Geometry check sheet. Reference: the model listing, model coordinates, mm. Coordinates: 2 decimals unless noted, no trailing zeros. Write each loop counter-clockwise with the first axis right and the second up, starting at its lowest first coordinate (ties: lowest second). Pieces come first, ordered by that corner, then holes. Notation, with made-up numbers: (35, 63) -> (76, 63) arc R17 cw to (76, 84) -> close; hole circle Ø7 at (20, 56). An arc over 180 degrees is marked (long way). Answer in a Markdown table with one row per item. Add a question column.
1. Cross-section at B-B on x = 17.5. Record the cut outline in (y, z), and give its area (3 significant figures).
2. Depth check by flat-ended pin: P1, Ø1.6, axis at x = 17.5, y = -52.5, coming from the -Z side. Enter the tip coordinate at first touch or a pass-through.
3. Scan line: L1, parallel to Y at x = 7.5, z = 6. Record every from-to range of solid material in increasing order. Write a range as from..to.
4. Cross-section at A-A on y = -7.5. Record the cut outline in (x, z), and give its area (3 significant figures).
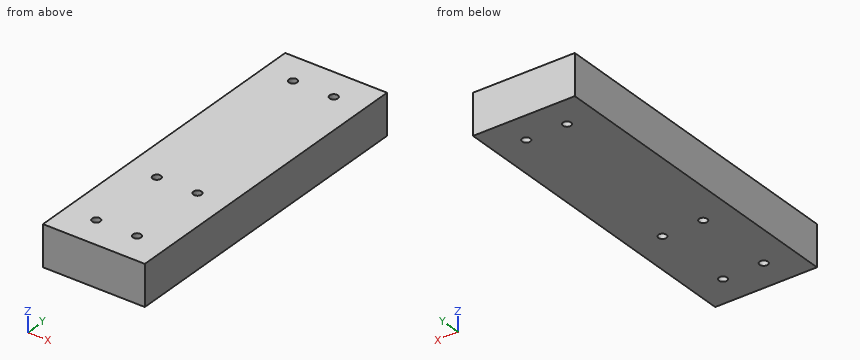
```python
from build123d import *

# Parameters (mm, degrees)
SKETCH1_W           = 25
SKETCH1_H           = 80
BOSS_EXTRUDE1_DEPTH = 10
SKETCH2_R           = 1
CUT_EXTRUDE1_DEPTH  = 85.409715081


with BuildPart() as part:
    # Sketch1 → Boss-Extrude1 (new body)
    with BuildSketch(Plane.XY):
        with Locations((12.5, -40)):
            Rectangle(SKETCH1_W, SKETCH1_H)
    extrude(amount=BOSS_EXTRUDE1_DEPTH)

    # Sketch2 → Cut-Extrude1 (cut, through all)
    with BuildSketch(Plane.XY.offset(10)):
        with Locations((7.5, -52.5)):
            Circle(SKETCH2_R)
        with Locations((7.5, -72.5)):
            Circle(SKETCH2_R)
        with Locations((7.5, -7.5)):
            Circle(SKETCH2_R)
        with Locations(Location((17.5, -7.5, 0), (0, 0, 180))):
            Circle(SKETCH2_R)
        with Locations(Location((17.5, -52.5, 0), (0, 0, 180))):
            Circle(SKETCH2_R)
        with Locations(Location((17.5, -72.5, 0), (0, 0, 180))):
            Circle(SKETCH2_R)
    extrude(amount=-CUT_EXTRUDE1_DEPTH, mode=Mode.SUBTRACT)


solid = part.part
```
Results found:
| question | item | result |
|---|---|---|
| 1 | outline | (-80, 0) -> (-73.5, 0) -> (-73.5, 10) -> (-80, 10) -> close; (-71.5, 0) -> (-53.5, 0) -> (-53.5, 10) -> (-71.5, 10) -> close; (-51.5, 0) -> (-8.5, 0) -> (-8.5, 10) -> (-51.5, 10) -> close; (-6.5, 0) -> (0, 0) -> (0, 10) -> (-6.5, 10) -> close |
| 1 | area | 740 mm^2 |
| 2 | P1 | passes through |
| 3 | L1 | y = -80..-73.5, -71.5..-53.5, -51.5..-8.5, -6.5..0 |
| 4 | outline | (0, 0) -> (6.5, 0) -> (6.5, 10) -> (0, 10) -> close; (8.5, 0) -> (16.5, 0) -> (16.5, 10) -> (8.5, 10) -> close; (18.5, 0) -> (25, 0) -> (25, 10) -> (18.5, 10) -> close |
| 4 | area | 210 mm^2 |
